```python
from build123d import *

# Parameters (mm, degrees)
BOSS_EXTRUDE1_DEPTH      = 5.5
BOSS_EXTRUDE1_DEPTH_BACK = 5.5
SKETCH1_W                = 42
SKETCH1_H                = 3
SKETCH2_OUTSIDE_W        = 52.704
SKETCH2_OUTSIDE_H        = 21.704
CUT_EXTRUDE1_DEPTH       = 28.717323103
BOSS_EXTRUDE2_DEPTH      = 10
BOSS_EXTRUDE2_DEPTH_BACK = 10
SKETCH3_R                = 0.5


with BuildPart() as part:
    # Sketch1 → Boss-Extrude1 (new, two sides: drawn at the far end of the back side and taken through both)
    with BuildSketch(Plane.XY.offset(-BOSS_EXTRUDE1_DEPTH_BACK)):
        with Locations((-6, 0)):
            Rectangle(SKETCH1_W, SKETCH1_H)
    extrude(amount=BOSS_EXTRUDE1_DEPTH + BOSS_EXTRUDE1_DEPTH_BACK)

    # Sketch2 outside → Cut-Extrude1 (cut, through all)
    with BuildSketch(Plane(origin=(0, 1.5, 0), x_dir=(1, 0, 0), z_dir=(0, 1, 0))):
        with Locations((-6, 0)):
            Rectangle(SKETCH2_OUTSIDE_W, SKETCH2_OUTSIDE_H)
        with BuildLine():
            Line((15, -4.25), (15, 4.25))
            Line((15, 4.25), (-17.478927243, 4.25))
            add(Edge.make_bspline(
                [(-17.478927243, 4.25), (-21.629138445, 5.5), (-27, 5.5)],
                knots=[0.883126675, 0.883126675, 0.883126675, 1.570796327, 1.570796327, 1.570796327], degree=2, weights=[1, 0.941468872, 1]))
            Line((-27, 5.5), (-27, -5.5))
            add(Edge.make_bspline(
                [(-27, -5.5), (-21.629138445, -5.5), (-17.478927243, -4.25)],
                knots=[4.71238898, 4.71238898, 4.71238898, 5.400058632, 5.400058632, 5.400058632], degree=2, weights=[1, 0.941468872, 1]))
            Line((-17.478927243, -4.25), (15, -4.25))
        make_face(mode=Mode.SUBTRACT)
    extrude(amount=-CUT_EXTRUDE1_DEPTH, mode=Mode.SUBTRACT)

    # Sketch3 → Boss-Extrude2 (add, two sides: drawn at the far end of the back side and taken through both)
    with BuildSketch(Plane.XY.offset(-BOSS_EXTRUDE2_DEPTH_BACK)):
        Circle(SKETCH3_R)
    extrude(amount=BOSS_EXTRUDE2_DEPTH + BOSS_EXTRUDE2_DEPTH_BACK)


solid = part.part
```
The model under review builds one solid part; all positions refer to its coordinate system, in mm. A direction names the side the tool comes from. Round coordinates to 2 decimals unless told otherwise and drop trailing zeros. Order: outer loops, then holes, each group sorted by start corner. A loop starts at its lowest first (then second) coordinate and runs counter-clockwise, first axis right, second up. Notation, with made-up numbers: M -23,64.25 L 8,64.25 A17 ccw 8,90.25 Z; hole C 37.5,3 d8. An arc over 180 degrees is marked long. Use a Markdown table: item, result.
1) Insertion check: pin 1 (1.5 mm diameter, centred on x = -8.5, y = 0.5, fed in from +Z). The pin has a flat end and moves straight along its axis. Give the tip position at first contact, or say it passes through.
Report:
| item | result |
|---|---|
| pin 1 | z = 4.25 |
2) Wall thickness on line 1 along Z through (x, y) = (-11.5, 1.15); line 2 along X through (y, z) = (-0.4, 9.25); line 3 along Z through (x, y) = (-20, 0.9): over which ranges is each line inside the solid? List them lowest first. Write a range as [from, to].
Report:
| item | result |
|---|---|
| line 1 | [-4.25, 4.25] |
| line 2 | [-0.3, 0.3] |
| line 3 | [-4.86, 4.86] |
3) Consider section B-B (z = 7.5). Write out the cut boundary in (x, y).
Report:
| item | result |
|---|---|
| outline | C 0,0 d1 |
4) Consider section A-A (x = 0). Write out the cut boundary in (y, z).
Report:
| item | result |
|---|---|
| outline | M -1.5,-4.25 L -0.5,-4.25 L -0.5,-10 L 0.5,-10 L 0.5,-4.25 L 1.5,-4.25 L 1.5,4.25 L 0.5,4.25 L 0.5,10 L -0.5,10 L -0.5,4.25 L -1.5,4.25 Z |
5) Draft analysis for pull direction X (two halves, no side actions). For faces 1 (the face through (-27, 0, 0)), 2 (the face through (-1, 0, 4.25)), 3 (the face through (0, 0, -10)), state which applies: released by +X, released by -X, zero draft, split by the parting line, or undercut.
Report:
| item | result |
|---|---|
| face 1 | released by -X |
| face 2 | undercut |
| face 3 | zero draft |
6) Tool access review of faces 4 (the face through (-0.108, -0.488, 7.085)), 5 (the face through (-0.108, -0.488, -7.165)), 6 (the face through (-6, 1.5, 0)): name each direction out of +Z, -Z, +X, -X, +Y, -Y from which nothing blocks a thin tool from reaching the whole face with its end or side.
Report:
| item | result |
|---|---|
| face 4 | +Z |
| face 5 | -Z |
| face 6 | +Z, -Z, +X, -X, +Y |
